Answer from the drawing. Dimensions are ordinates in mm from the lowest x, y and z of the part. Give positions to 0.01 mm unless a question says otherwise; leave off trailing zeros. Loops run counter-clockwise (first coordinate to the right, second up) from the corner with the lowest first, then second, coordinate; pieces in that order, holes last.
(1) Find section A-A, the plane z = 26. Write down the section's boundary in (x, y).
(2) Find section B-B, the plane y = 1.4. State how many separate pieces and enclosed holes the cut face has, then the cut area to 3 significant figures.
(3) Each of these flat-tipped pins is pushed along its axis until it touches: P1, Ø0.6, axis at x = 11.5, y = 1, coming from the -Z side; P2, Ø0.6, axis at y = 0.5, z = 12.5, coming from the -X side; P3, Ø0.6, axis at x = 28, y = 0.5, coming from the +Z side. Where does it stop, or does it pass through?
(4) Straight lines are drawn through the part: probe 1 along X at (y, z) = (0.5, 21.5) (3 decimals); probe 2 along X at (y, z) = (1.95, 24.5); probe 3 along X at (y, z) = (0.2, 61). For each, find the intervals that lie inside material, in ascending order.
(5) Find section C-C, the plane z = 60.5. Write down the section's boundary in (x, y).
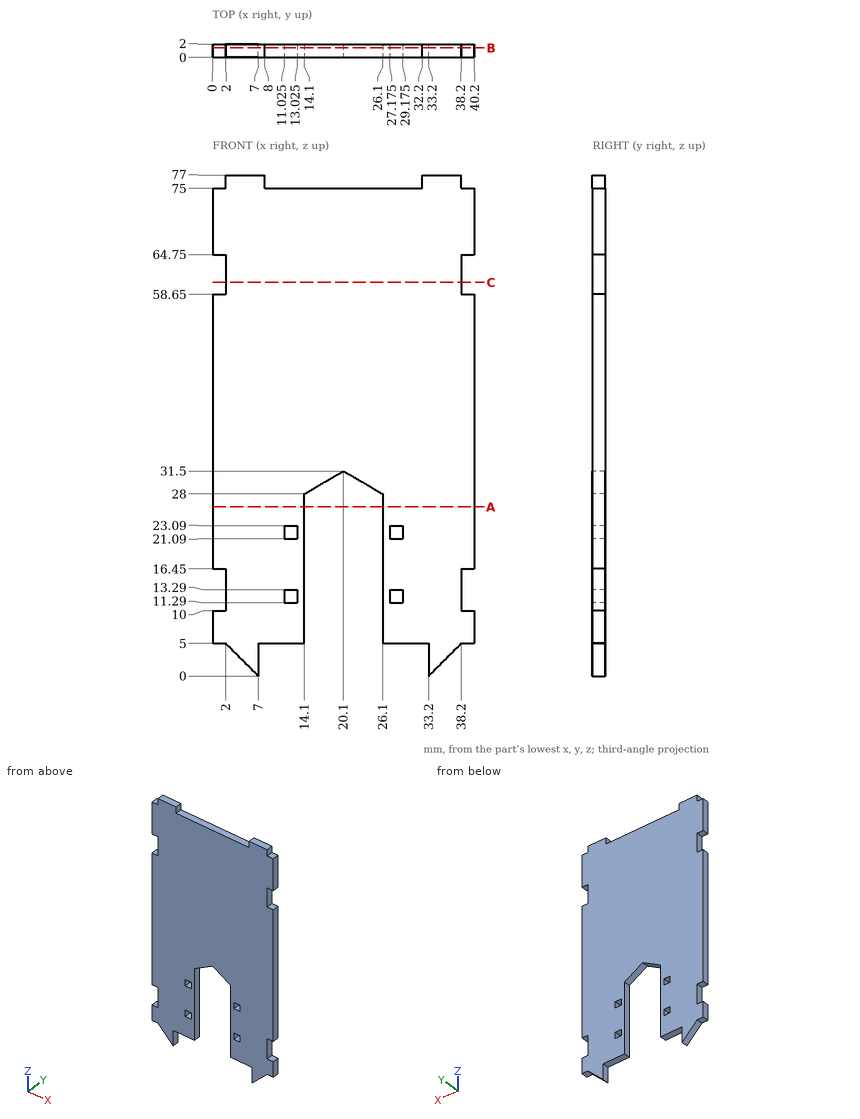
Entries:
1. outline: (0, 0) - (14.1, 0) - (14.1, 2) - (0, 2) - close; (26.1, 0) - (40.2, 0) - (40.2, 2) - (26.1, 2) - close
2. separate pieces: 1
2. enclosed holes: 4
2. area: 2,500 mm2
3. P1: stops at z = 5
3. P2: stops at x = 2
3. P3: stops at z = 75
4. probe 1: x = 0 to 11.025, 13.025 to 14.1, 26.1 to 27.175, 29.175 to 40.2
4. probe 2: x = 0 to 14.1, 26.1 to 40.2
4. probe 3: x = 2 to 38.2
5. outline: (2, 0) - (38.2, 0) - (38.2, 2) - (2, 2) - close
